Study the drawing (mm; zero at the part's minimum x, y, z) and answer. A direction names the side the tool comes from. Round coordinates to 2 decimals unless told otherwise and drop trailing zeros. Write each loop counter-clockwise with the first axis right and the second up, starting at its lowest first coordinate (ties: lowest second). Pieces come first, ordered by that corner, then holes. Notation, with made-up numbers: (-36, -4) - (1, -4) arc R23 ccw to (1, 28) - close; hole circle Ø10 at (71.5, 86.5). An arc over 180 degrees is marked (long way). Use one line per item in the form item = value. Start each with the question number.
1) For a pull along Y with two mould halves and no side action, classify the marked faces 1, 2, 3 and 4 as released by +Y, released by -Y, zero draft, split by the parting line, or undercut.
2) The part is cut by section D-D, the plane y = 11.75. Give the vertices of the cut face in (x, z).
3) The part is cut by section C-C, the plane x = 7.1. Give the vertices of the cut face in (y, z), plus the area to 3 significant figures.
4) The part is cut by section A-A, the plane y = 7.05. Give the vertices of the cut face in (x, z).
5) Each of these flat-tipped pins is pushed along its axis until it touches: pin 1 (1.8 mm diameter, centred on x = 28.5, y = 7.5, fed in from +Z); pin 2 (5 mm diameter, centred on y = 8.5, z = 8, fed in from -X); pin 3 (8 mm diameter, centred on x = 21, y = 2, fed in from +Z). Where does it stop, or does it pass through?
6) The part is cut by section B-B, the plane z = 1. Give the vertices of the cut face in (x, y).
7) Consider line 1 along Y through (x, z) = (7.1, 1); line 2 along X through (y, z) = (10.25, 9.5); line 3 along Z through (x, y) = (23, 7.75). Determine where each line is inside the solid, lowest interval first. Write a range as from..to.
8) For the marked faces 5 and 6, determine the directions among +Z, -Z, +X, -X, +Y, -Y from which every point of the face is accessible in a straight line to the end or side of a thin tool.
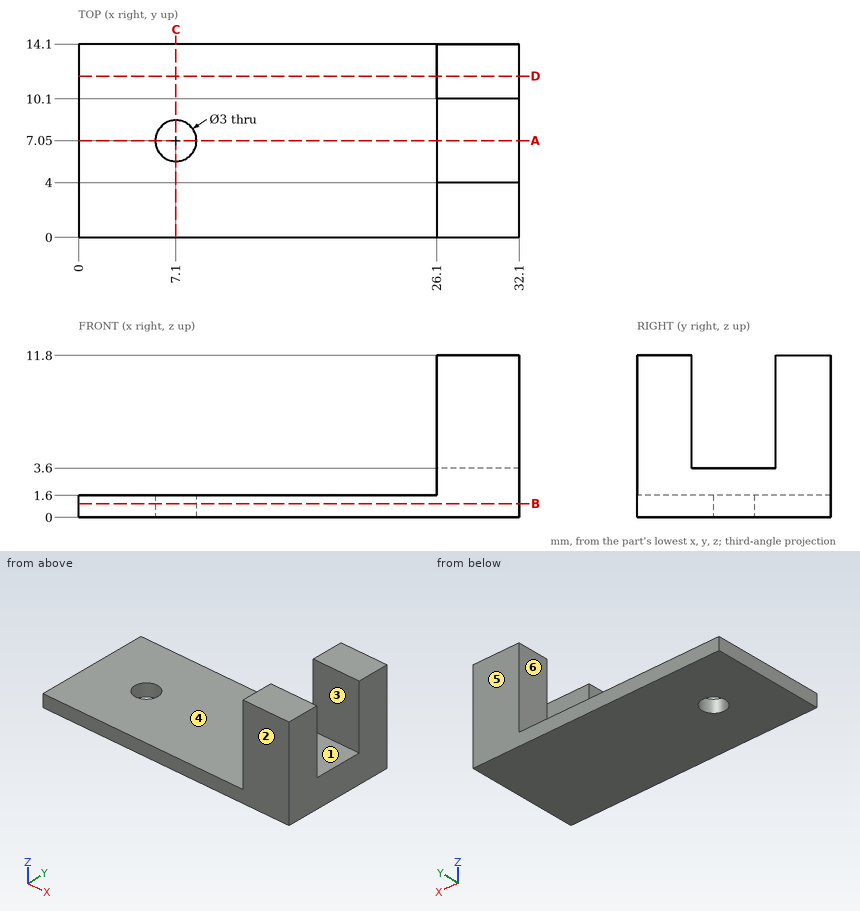
Geometry results:
q1.face_1 = undercut
q1.face_2 = released by -Y
q1.face_3 = undercut
q1.face_4 = zero draft
q2.outline = (0, 0) - (32.1, 0) - (32.1, 11.8) - (26.1, 11.8) - (26.1, 1.6) - (0, 1.6) - close
q3.outline = (0, 0) - (5.55, 0) - (5.55, 1.6) - (0, 1.6) - close; (8.55, 0) - (14.1, 0) - (14.1, 1.6) - (8.55, 1.6) - close
q3.area = 17.8 mm2
q4.outline = (0, 0) - (5.6, 0) - (5.6, 1.6) - (0, 1.6) - close; (8.6, 0) - (32.1, 0) - (32.1, 3.6) - (26.1, 3.6) - (26.1, 1.6) - (8.6, 1.6) - close
q5.pin_1 = 3.6
q5.pin_2 = 26.1
q5.pin_3 = 1.6
q6.outline = (0, 0) - (32.1, 0) - (32.1, 14.1) - (0, 14.1) - close; hole circle Ø3 at (7.1, 7.05)
q7.line_1 = 0..5.55, 8.55..14.1
q7.line_2 = 26.1..32.1
q7.line_3 = 0..1.6
q8.face_5 = +Z, -Z, +X, -X, +Y
q8.face_6 = +Z, -X, +Y, -Y
